from build123d import *

# Parameters (mm, degrees)
F3_DEPTH = 560
F4_DEPTH = 100


with BuildPart() as f3:
    # F2 (on Right) → F3 (new body)
    with BuildSketch(Plane.YZ):
        with BuildLine():
            Line((-70, -300), (400, -300))
            Line((400, -300), (400, 300))
            Line((400, 300), (-400, 300))
            Line((-400, 300), (-400, -300))
            Line((-400, -300), (-330, -300))
            ThreePointArc((-330, -300), (-200, -170), (-70, -300))
        make_face()
        with BuildLine():
            Line((-330, -300), (-70, -300))
            ThreePointArc((-70, -300), (-200, -170), (-330, -300))
        make_face()
    extrude(amount=F3_DEPTH)

    # F2 (on Right) → F4 (join)
    with BuildSketch(Plane.YZ):
        with BuildLine():
            ThreePointArc((-330, -300), (-200, -430), (-70, -300))
            Line((-70, -300), (-330, -300))
        make_face()
        with BuildLine():
            Line((-330, -300), (-70, -300))
            ThreePointArc((-70, -300), (-200, -170), (-330, -300))
        make_face()
    extrude(amount=-F4_DEPTH)

    # F6: F3 across plane


with BuildPart() as f3_1:
    add(f3.part)
    add(f3.part.mirror(Plane(origin=(300, 11.7085678948, 14.3328259835), x_dir=(0, 1, 0), z_dir=(-1, 0, 0))))


solid = f3_1.part
Work out the finished part from the listing and answer in its coordinate system (mm). A direction names the side the tool comes from. Give positions to 0.01 mm unless a question says otherwise; leave off trailing zeros. Write each loop counter-clockwise with the first axis right and the second up, starting at its lowest first coordinate (ties: lowest second). Pieces come first, ordered by that corner, then holes. Notation, with made-up numbers: (87, 48.5) - (123, 48.5) arc R37 cw to (123, 84.5) - close; hole circle Ø11 at (75, 80.5). An arc over 180 degrees is marked (long way). One line per item, written item: value. Start each with the question number.
1. Find section A-A (y = -200). Write down the section's boundary in (x, z).
2. Consider probe 1 along X at (y, z) = (351, -97); probe 2 along Z at (x, y) = (524, 329.5); probe 3 along Z at (x, y) = (-43, -129.5). Determine where each line is inside the solid, lowest interval first.
3. Given pin 1 (5 mm diameter, centred on x = 64.5, y = 273, fed in from -Z); pin 2 (8 mm diameter, centred on y = 169.5, z = -184, fed in from +X), each flat-ended and moving along its own axis, determine where each tip first touches the part or whether it passes through.
4. Find section C-C (x = 491.5). Write down the section's boundary in (y, z).
5. Find section B-B (z = 249). Write down the section's boundary in (x, y).
6. Find section D-D (z = -285.5). Write down the section's boundary in (x, y), then the cut area to 3 significant figures.
7. For faces 1 (the flat face through (304, 6, 300)), 2 (the flat face through (304, -400, 4)), 3 (the cylindrical face through (-49.3, -216.923, -171.106)), 4 (the flat face through (600, -202, -350)), 5 (the cylindrical face through (649.3, -216.923, -171.106)), determine the directions among +Z, -Z, +X, -X, +Y, -Y from which every point of the face is accessible in a straight line to the end or side of a thin tool.
Geometry results:
1. outline: (-100, -430) - (0, -430) - (0, -300) - (600, -300) - (600, -430) - (700, -430) - (700, -170) - (600, -170) - (600, 300) - (0, 300) - (0, -170) - (-100, -170) - close
2. probe 1: 0 to 600
2. probe 2: -300 to 300
2. probe 3: -409.22 to -190.78
3. pin 1: z = -300
3. pin 2: x = 600
4. outline: (-400, -300) - (400, -300) - (400, 300) - (-400, 300) - close
5. outline: (0, -400) - (600, -400) - (600, 400) - (0, 400) - close
6. outline: (-100, -329.19) - (0, -329.19) - (0, -400) - (600, -400) - (600, -329.19) - (700, -329.19) - (700, -70.81) - (600, -70.81) - (600, 400) - (0, 400) - (0, -70.81) - (-100, -70.81) - close
6. area: 532,000 mm2
7. face 1: +Z, +X, -X, +Y, -Y
7. face 2: +Z, -Z, +X, -X, -Y
7. face 3: -X
7. face 4: -Z, +Y, -Y
7. face 5: +X
